Here's how the part is built. I have some questions about the finished solid (model axes, mm). A direction names the side the tool comes from. Round coordinates to 2 decimals unless told otherwise and drop trailing zeros. Write each loop counter-clockwise with the first axis right and the second up, starting at its lowest first coordinate (ties: lowest second). Pieces come first, ordered by that corner, then holes. Notation, with made-up numbers: (20, 17) - (52, 17) arc R21 ccw to (52, 22) - close; hole circle Ø8 at (60.5, -22.75). An arc over 180 degrees is marked (long way). Write item = value, one per line. Start each with the question number.
Item 1: If we section it at A-A (y = 82.5): Give the number of separate pieces and of enclosed holes in the cut face, and give its area (3 significant figures).
Item 2: If we section it at D-D (z = 38): Please give me the cut outline in (x, y).
Item 3: Thinking about a two-plate mould opening in Z: for faces 6 (the face through (20, 0, 53)), 7 (the face through (12, 6.35, 63)), 8 (the face through (58.67, 43.68, 48.44)), 9 (the face through (56, 71.068, 56)), which applies, pulls with the +Z half, pulls with the -Z half, needs draft (parallel to the pull), parting line crosses it, or undercut?
Item 4: If I drill on line 1 along Y through (x, z) = (14, 64.5); line 2 along Z through (x, y) = (-13, 66); line 3 along Z through (x, y) = (31, 20.5), over which ranges is the centre line in solid material (lowest first)? Write a range as [from, to].
Item 5: Which directions (+Z, -Z, +X, -X, +Y, -Y) give clear straight access to the entire face, cutting with the end or side of a thin tool? Please do faces 1 (the face through (17, 88.594, 50)), 2 (the face through (15.15, 73.57, 51.18)), 3 (the face through (24.89, 8.18, 78.18)), 4 (the face through (8.463, 3.131, 54.372)), 5 (the face through (66, 66.517, 57)).
Item 6: For P1, Ø1, axis at y = 40.5, z = 62, coming from the -X side; P2, Ø6, axis at x = 58.5, z = 66.5, coming from the -Y side; P3, Ø5.5, axis at x = 10, z = 62, coming from the -Y side, each with a flat end and sliding along its axis, tell me the tip position at first contact or that it passes through.
Item 7: If we section it at B-B (x = 25): Please give me the cut outline in (y, z).
```python
from build123d import *

# Parameters (mm, degrees)
BOSS_EXTRUDE1_DEPTH          = 88.5939681
CUT_EXTRUDE5_DEPTH           = 30.48
SKETCH13_W                   = 39.37
SKETCH13_H                   = 27.94
CUT_EXTRUDE6_DEPTH           = 121.173808566
SKETCH17_W                   = 9.779
SKETCH17_H                   = 16.129
SKETCH20_W                   = 22.076995977
SKETCH20_H                   = 19.05
BOSS_EXTRUDE2_DEPTH          = 43.18
CUT_EXTRUDE9_START           = -22.076995977
CUT_EXTRUDE9_DEPTH           = 22.076995977
FILLET2_R                    = 2.54
CUT_EXTRUDE11_DEPTH          = 150.440180481
F_10_0_1935_DIAMETER_HOLE1_D = 4.9149
CUT_EXTRUDE14_DEPTH          = 12.7
FILLET5_R                    = 2.54
SKETCH31_RX                  = 22.225
SKETCH31_RY                  = 6.35
CUT_EXTRUDE16_DEPTH          = 150.440180481
FILLET6_R                    = 2.54
SKETCH32_R                   = 9.525
CUT_EXTRUDE17_DEPTH          = 6.35


# Read off the part's stored shape, not the designer's step: Cut-Extrude9
with BuildPart() as part:
    # Sketch1 → Boss-Extrude1 (new body)
    with BuildSketch(Plane(origin=(0, 0, 0), x_dir=(1, 0, 0), z_dir=(0, 1, 0))):
        with BuildLine():
            Line((63.017839503, -66.782093), (53.468205472, -26.506342671))
            Line((53.468205472, -26.506342671), (-35.875703335, -47.690346072))
            Line((-35.875703335, -47.690346072), (-26.326069304, -87.966096401))
            ThreePointArc((-26.326069304, -87.966096401), (21.184003401, -89.343908807), (63.017839503, -66.782093))
        make_face()
    extrude(amount=BOSS_EXTRUDE1_DEPTH)

    # Sketch12 → Cut-Extrude5 (cut)
    with BuildSketch(Plane(origin=(0, 88.5939681, 0), x_dir=(1, 0, 0), z_dir=(0, 1, 0))):
        Polygon((5.316172436, -88.753304237), (43.624072478, -79.670259902), (35.713033863, -46.305314704), (-2.594866179, -55.388359039), align=None)
    extrude(amount=-CUT_EXTRUDE5_DEPTH, mode=Mode.SUBTRACT)

    # Sketch13 → Cut-Extrude6 (cut, through all)
    with BuildSketch(Plane(origin=(20.206823904, 0, 85.222637004), x_dir=(-0.9730226071044289, 0, 0.23070978753338656), z_dir=(-0.23070978753338653, 0, -0.9730226071044288))):
        with Locations((-4.3815, 74.6239681)):
            Rectangle(SKETCH13_W, SKETCH13_H)
    extrude(amount=-CUT_EXTRUDE6_DEPTH, mode=Mode.SUBTRACT)

    # Sketch17 → Cut-Revolve1 (revolve, cut)
    with BuildSketch(Plane(origin=(0, 0, 0), x_dir=(0.2779727925443418, 0, 0.9605889477841708), z_dir=(-0.9605889477841708, 0, 0.2779727925443418))):
        with Locations((86.934262311, 8.0645)):
            Rectangle(SKETCH17_W, SKETCH17_H)
    revolve(axis=Axis((0, 88.5939681, 0), (0, -1, 0)), mode=Mode.SUBTRACT)

    # Sketch20 → Boss-Extrude2 (add)
    with BuildSketch(Plane(origin=(46.161246838, 0, 1.33869588), x_dir=(0, -1, 0), z_dir=(0.9995797526704859, 0, 0.02898823987775881))):
        with Locations((-77.555470112, -56.021383933)):
            Rectangle(SKETCH20_W, SKETCH20_H)
    extrude(amount=BOSS_EXTRUDE2_DEPTH)

    # Cut-Extrude9 outline → Cut-Extrude9 (cut)
    with BuildSketch(Plane(origin=(0, 88.5939681, 0), x_dir=(1, 0, 0), z_dir=(0, 1, 0)).offset(CUT_EXTRUDE9_START)):
        with BuildLine():
            Line((87.975252227, -49.06725203), (77.797045472, -48.772079686))
            ThreePointArc((77.797045472, -48.772079686), (70.701096399, -58.587123236), (62.37506144, -67.382844638))
            Line((62.37506144, -67.382844638), (87.423026258, -68.109246318))
            Line((87.423026258, -68.109246318), (87.975252227, -49.06725203))
        make_face()
    extrude(amount=CUT_EXTRUDE9_DEPTH, mode=Mode.SUBTRACT)

    # Fillet2
    fillet2_edges = [part.edges().sort_by_distance(p)[0] for p in [
        (68.206351325, 66.516972123, 48.493945458),
        (68.206351325, 88.5939681, 48.493945458),
        (-35.875703335, 44.29698405, 47.690346072),
        (53.468205472, 44.29698405, 26.506342671),
    ]]
    fillet(fillet2_edges, radius=FILLET2_R)

    # Sketch25 → Cut-Extrude11 (cut, through all)
    with BuildSketch(Plane.XZ):
        Polygon((-24.667480264, 53.125115211), (-13.767913037, 99.094232658), (-26.000188569, 101.994582217), (-40.190153369, 42.148154842), (65.286931214, 17.138873869), (68.442798797, 30.762859127), align=None)
    extrude(amount=-CUT_EXTRUDE11_DEPTH, mode=Mode.SUBTRACT)

    # #10 (0.1935) Diameter Hole1 (through all)
    with Locations(Plane(origin=(0, 0, 0), x_dir=(-1, 0, 0), z_dir=(0, -1, 0))):
        with Locations((10.85357172, -56.338005803), (-32.898719503, -44.680648661)):
            Hole(F_10_0_1935_DIAMETER_HOLE1_D / 2)

    # Sketch30 → Cut-Extrude14 (cut)
    with BuildSketch(Plane(origin=(0, 71.0679681, 0), x_dir=(1, 0, 0), z_dir=(0, 1, 0))):
        Polygon((30.706346029, -52.713276699), (36.885039584, -51.248269548), (81.505966291, -52.542295486), (81.257041939, -61.125767384), (38.936049595, -59.898440526), (32.75735604, -61.363447676), align=None)
    extrude(amount=CUT_EXTRUDE14_DEPTH, mode=Mode.SUBTRACT)

    # Fillet5
    fillet5_edges = [part.edges().sort_by_distance(p)[0] for p in [
        (55.229871942, 44.29698405, 33.936202145),
    ]]
    fillet(fillet5_edges, radius=FILLET5_R)

    # Sketch31 → Cut-Extrude16 (cut, through all)
    with BuildSketch(Plane.XZ):
        with Locations(Location((-24.667480264, 53.125115211), (0, 0, 76.661136503))):
            Ellipse(SKETCH31_RX, SKETCH31_RY)
    extrude(amount=-CUT_EXTRUDE16_DEPTH, mode=Mode.SUBTRACT)

    # Fillet6
    fillet6_edges = [part.edges().sort_by_distance(p)[0] for p in [
        (-18.49303476, 44.29698405, 51.642201263),
        (-19.539955236, 44.29698405, 74.750542654),
    ]]
    fillet(fillet6_edges, radius=FILLET6_R)

    # Sketch32 → Cut-Extrude17 (cut)
    with BuildSketch(Plane.XZ):
        with Locations(Location((12.111377962, 63.170347591, 0), (0, 0, 270))):
            Circle(SKETCH32_R)
    extrude(amount=-CUT_EXTRUDE17_DEPTH, mode=Mode.SUBTRACT)


solid = part.part
```
Reply:
q1.separate_pieces = 2
q1.enclosed_holes = 1
q1.area = 1,760 mm2
q2.outline = (38.31, 0) - (56.19, 0) - (56.19, 88.59) - (38.31, 88.59) - close
q3.face_6 = needs draft
q3.face_7 = undercut
q3.face_8 = pulls with the -Z half
q3.face_9 = undercut
q4.line_1 = [6.35, 58.11]
q4.line_2 = [50.32, 55.14], [57.53, 90.9]
q4.line_3 = [39.76, 43.12], [46.24, 86.43]
q5.face_1 = +Z, -Z, +X, -X, +Y
q5.face_2 = +Y
q5.face_3 = +Z, -Y
q5.face_4 = -Y
q5.face_5 = -Z, +X, -Y
q6.P1 = -16.85
q6.P2 = 16.13
q6.P3 = 6.35
q7.outline = (0, 41.2) - (88.59, 41.2) - (88.59, 48.85) - (58.11, 48.85) - (58.11, 84.09) - (60.65, 84.09) - (60.65, 88.35) - (16.13, 88.35) - (16.13, 78.14) - (0, 78.14) - close
